Autodesk Fusion 360 part; units mm, degrees
sketch "Sketch1" plane through (0, 0, 0) normal (0, 0, 1) x (1, 0, 0)
  line L0 (0, 0) -> (-122.75, 0) construction
  line L1 (0, 0) -> (0, 25.25) construction
  line L2 (0, 0) -> (122.75, 0) construction
  line L3 (0, 0) -> (0, -25.25) construction
  circle A0 centre (-122.75, 0) radius 2.5
  circle A1 centre (122.75, 0) radius 2.5
  line L4 (-57, 25.5) -> (57, 25.5)
  line L5 (57, 25.5) -> (57, -25.5)
  line L6 (57, -25.5) -> (-57, -25.5)
  line L7 (-57, -25.5) -> (-57, 25.5)
  line L8 (-57, 25.5) -> (57, -25.5) construction
  line L9 (57, 25.5) -> (-57, -25.5) construction
  line L10 (-117.75, 5) -> (-127.75, 5)
  line L11 (-127.75, 5) -> (-127.75, -5)
  line L12 (-127.75, -5) -> (-117.75, -5)
  line L13 (-117.75, -5) -> (-117.75, 5)
  line L14 (-117.75, 5) -> (-127.75, -5) construction
  line L15 (-127.75, 5) -> (-117.75, -5) construction
  line L16 (-117.75, 5) -> (-57, 5)
  line L17 (-57, 5) -> (-57, -5)
  line L18 (-57, -5) -> (-117.75, -5)
  line L19 (-117.75, -5) -> (-117.75, 5)
  line L20 (117.75, -5) -> (117.75, 5)
  line L21 (127.75, 5) -> (127.75, -5)
  line L22 (117.75, 5) -> (127.75, -5) construction
  line L23 (117.75, -5) -> (117.75, 5)
  line L24 (127.75, 5) -> (117.75, -5) construction
  line L25 (127.75, -5) -> (117.75, -5)
  line L26 (117.75, 5) -> (127.75, 5)
  circle A2 centre (122.75, 0) radius 2.5
  line L27 (117.75, 5) -> (57, 5)
  line L28 (57, -5) -> (117.75, -5)
  line L29 (59, 27.5) -> (-59, 27.5)
  line L30 (-59, 27.5) -> (-59, -27.5)
  line L31 (-59, -27.5) -> (59, -27.5)
  line L32 (59, -27.5) -> (59, 27.5)
  line L33 (59, 27.5) -> (-59, -27.5) construction
  line L34 (-59, 27.5) -> (59, -27.5) construction
  point P0 (-122.75, 0)
  point P1 (122.75, 0)
  point P2 (122.75, 0)
  dimension "d1" = 122.75
  dimension "d2" = 25.25
  dimension "d3" = 5
  dimension "d4" = 114
  dimension "d5" = 51
  dimension "d6" = 10
  dimension "d7" = 10
  dimension "d8" = 10
  dimension "d19" = 118
  dimension "d20" = 55
extrude "Extrude2" add sketch "Sketch1" along normal blind 10 contours L10 L11 L12 L13 L19 | L20 L21 L23 L25 L26 makes body 1 at (125.2469, -0.1246, 6.6667) makes body 2 at (-120.2531, -0.1246, 6.6667)
sketch "Sketch2" plane through (0, 5, 0) normal (0, 1, 0) x (-1, 0, 0)
  line L0 (117.75, 0) -> (127.75, 0)
  line L1 (127.75, 0) -> (127.75, 10)
  line L2 (127.75, 10) -> (117.75, 10)
  arc A0 (57, 100) -> (117.75, 10) centre (154.0417, 100) ccw
  line L3 (117.75, 10) -> (117.75, 0)
sketch "Sketch3" plane through (0, 5, 0) normal (0, 1, 0) x (-1, 0, 0)
  line L0 (-127.75, 0) -> (-117.75, 0)
  line L1 (-117.75, 10) -> (-127.75, 10)
  line L2 (-127.75, 10) -> (-127.75, 0)
  arc A0 (-117.75, 10) -> (-57, 100) centre (-154.0417, 100) ccw
  line L3 (-117.75, 0) -> (-117.75, 10)
extrude "Extrude7" add sketch "Sketch1" along normal blind 100 separate body contours L4 L5 L7 L16 L27 L29 L30 L32 | L7 L16 L17 L18 L30 | L5 L27 L28 L32 | L5 L6 L7 L18 L28 L30 L31 L32 makes body 3
extrude "Extrude8" add sketch "Sketch1" along normal blind 100 contours L13 L16 L18 L19 L30 | L20 L23 L27 L28 L32 bodies 1 2 3
sketch "Sketch4" plane through (0, -5, 0) normal (0, -1, 0) x (1, 0, 0)
  line L0 (-127.75, 0) -> (-59, 0)
  line L1 (-59, 0) -> (-59, 100)
  line L2 (-59, 100) -> (-117.75, 100)
  line L3 (-117.75, 100) -> (-117.75, 10)
  line L4 (-117.75, 10) -> (-127.75, 10)
  line L5 (-127.75, 10) -> (-127.75, 0)
  arc A0 (-117.75, 10) -> (-59, 100) centre (-154.7515, 98.3291) ccw
sketch "Sketch5" plane through (0, -5, 0) normal (0, -1, 0) x (1, 0, 0)
  line L0 (59, 0) -> (127.75, 0)
  line L1 (127.75, 0) -> (127.75, 10)
  line L2 (127.75, 10) -> (117.75, 10)
  line L3 (117.75, 10) -> (117.75, 100)
  line L4 (117.75, 100) -> (59, 100)
  line L5 (59, 100) -> (59, 0)
  arc A0 (59, 100) -> (117.75, 10) centre (157.3112, 100) ccw
extrude "Extrude9" cut sketch "Sketch5" sketch "Sketch4" against normal blind 35 contours L3 L4 A0 of sketch 2 contours L1 L2 L3 A0 bodies 1
sketch "Sketch6" plane through (0, -27.5, 0) normal (0, -1, 0) x (1, 0, 0)
  line L0 (-59, 0) -> (59, 0)
  line L1 (59, 0) -> (59, 100)
  line L2 (59, 100) -> (-59, 100)
  line L3 (-59, 100) -> (-59, 0)
  line L4 (-45, 0) -> (45, 0) construction
  line L5 (45, 0) -> (45, 37.4909) construction
  line L6 (45, 37.4909) -> (-45, 37.4909) construction
  line L7 (-45, 37.4909) -> (-45, 0) construction
  line L8 (-45, 0) -> (45, 37.4909) construction
  line L9 (45, 0) -> (-45, 37.4909) construction
  arc A0 (45, 0) -> (-45, 0) centre (0, 1.4121) ccw
  point P0 (0, 18.7455)
  dimension "d29" = 90
extrude "Extrude10" cut sketch "Sketch6" against normal blind 95 contours L0 A0 bodies 1
sketch "Sketch7" plane through (-59, 0, 0) normal (-1, 0, 0) x (0, -1, 0)
  line L0 (-27.5, 100) -> (-27.5, 0)
  line L1 (-27.5, 0) -> (-5, 0)
  line L2 (-5, 0) -> (-5, 96.6583)
  line L3 (-5, 96.6583) -> (5, 96.6583)
  line L4 (5, 96.6583) -> (5, 0)
  line L5 (5, 0) -> (27.5, 0)
  line L6 (27.5, 0) -> (27.5, 100)
  line L7 (27.5, 100) -> (-27.5, 100)
  ellipse E0 centre (-16.1457, 25.858) end of major axis (-16.1457, 9.4792) minor radius 8.2129
  line L8 (-16.1457, 42.2368) -> (-16.1457, 9.4792) construction
  line L9 (-24.3586, 25.858) -> (-7.9328, 25.858) construction
  ellipse E1 centre (15.8543, 25.858) end of major axis (15.8543, 9.4792) minor radius 8.2129
  line L10 (15.8543, 42.2368) -> (15.8543, 9.4792) construction
  line L11 (7.6414, 25.858) -> (24.0672, 25.858) construction
  point P0 (-16.1457, 25.858)
extrude "Extrude11" cut sketch "Sketch7" against normal blind 145 contours E0 | E1 bodies 1
equation "d1 = ( 245.5 / 2 ) * 1 mm"
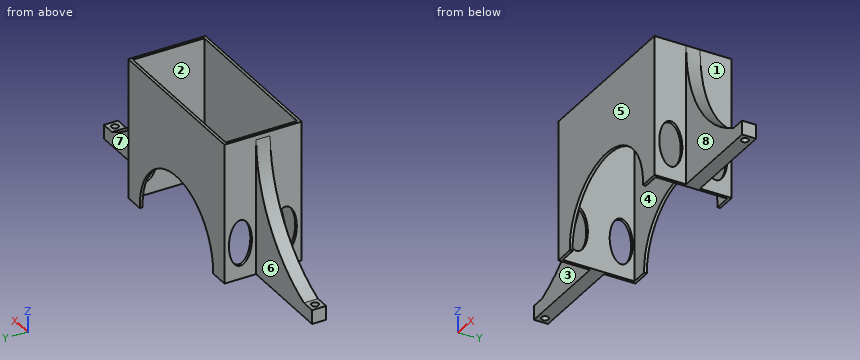
Verification items for the finished model (mm, model axes). Face numbers are marked on the shaded views. A direction names the side the tool comes from. Give positions to 0.01 mm unless a question says otherwise; leave off trailing zeros. Loops run counter-clockwise (first coordinate to the right, second up) from the corner with the lowest first, then second, coordinate; pieces in that order, holes last.
1) Sectioned sample at A-A, the plane x = 122.75. Enter the section's corners in (y, z), then the cut area to 3 significant figures.
2) Draft check along X on the marked faces 1, 2 and 3. Enter one of: pulls with the +X half, pulls with the -X half, needs draft (parallel to the pull), parting line crosses it, or undercut.
3) Depth check by flat-ended pin: pin 1 Ø2 at (y, z) = (9.5, 47) entering from +X; pin 2 Ø15.5 at (y, z) = (9, 35) entering from +X; pin 3 Ø8 at (x, y) = (-121.5, -1.5) entering from +Z. Enter the tip coordinate at first touch or a pass-through.
4) Sectioned sample at B-B, the plane y = 0. Enter the section's corners in (x, z).
5) Sectioned sample at C-C, the plane z = 82. Enter the section's corners in (x, y), then the cut area to 3 significant figures.
6) Thickness scan on line 1 along Y through (x, z) = (44, 59); line 2 along X through (y, z) = (25, 66); line 3 along Y through (x, z) = (-122.75, 4.75). Record the ranges inside material, lowest first.
7) Set-up check for the marked faces 4, 5, 6, 7 and 8: record each of +Z, -Z, +X, -X, +Y, -Y from which the full face is reachable in a straight line by a thin tool's end or side.
8) Sectioned sample at D-D, the plane x = -51. Enter the section's corners in (y, z).
Answers:
1. outline: (-5, 0) - (-2.5, 0) - (-2.5, 10) - (-5, 10) - close; (2.5, 0) - (5, 0) - (5, 10) - (2.5, 10) - close
1. area: 50.0 mm2
2. face 1: pulls with the +X half
2. face 2: undercut
2. face 3: needs draft
3. pin 1: stops at x = 59
3. pin 2: stops at x = 89.98
3. pin 3: stops at z = 10.11
4. outline: (-127.75, 0) - (-125.25, 0) - (-125.25, 10) - (-127.75, 10) - close; (-120.25, 0) - (-57, 0) - (-57, 100) - (-59, 100) - (-59, 96.66) arc R95.77 cw to (-117.75, 10) - (-120.25, 10) - close; (57, 0) - (120.25, 0) - (120.25, 10) - (117.75, 10) arc R98.31 cw to (59, 100) - (57, 100) - close; (125.25, 0) - (127.75, 0) - (127.75, 10) - (125.25, 10) - close
5. outline: (-60.39, -5) - (-59, -5) - (-59, -27.5) - (59, -27.5) - (59, -5) - (60.66, -5) - (60.66, 5) - (59, 5) - (59, 27.5) - (-59, 27.5) - (-59, 5) - (-60.39, 5) - close; hole (-57, -25.5) - (57, -25.5) - (57, 25.5) - (-57, 25.5) - close
5. area: 706 mm2
6. line 1: y = -27.5 to -25.5, 25.5 to 27.5
6. line 2: x = -59 to -57, 57 to 59
6. line 3: y = -5 to -2.5, 2.5 to 5
7. face 4: +Z, -Z
7. face 5: +Z, -Z, +X, -X, -Y
7. face 6: +Z, -Z, -X, +Y
7. face 7: +Z, -Z, +X, +Y
7. face 8: +Z, -Z, +X, -Y
8. outline: (-27.5, 0) - (-25.5, 0) - (-25.5, 100) - (-27.5, 100) - close; (25.5, 0) - (27.5, 0) - (27.5, 100) - (25.5, 100) - close
